Read the model definition and answer for the solid it produces. Units are mm, in the model's axes. Face numbers are marked on the shaded views. A direction names the side the tool comes from. Give positions to 0.01 mm unless a question says otherwise; leave off trailing zeros. Order: outer loops, then holes, each group sorted by start corner. A loop starts at its lowest first (then second) coordinate and runs counter-clockwise, first axis right, second up. Notation, with made-up numbers: (-17.5, 25) - (-5.5, 25) arc R24 cw to (-5.5, 42) - close; hole circle Ø3 at (39, 7.5). An arc over 180 degrees is marked (long way). Use a Markdown table: item, result. Add a question column.
1. Which of the six approach directions +Z, -Z, +X, -X, +Y, -Y give full straight-line access (tool end or side, diameter ignored) to the marked faces 1, 2, 3 and 4?
2. A cutting plane is placed at C-C on y = -30. Determine the outline of the cut face in (x, z), and give its area (3 significant figures).
3. A cutting plane is placed at A-A on x = 0. Determine the outline of the cut face in (y, z).
4. Flat-ended cylindrical pins translate along their axes: P1, Ø15, axis at y = -44, z = 15.5, coming from the +X side; P2, Ø24, axis at x = -49.5, y = -37.5, coming from the +Z side; P3, Ø24, axis at y = -34, z = 13, coming from the -X side; P4, Ø4, axis at x = -16, z = 19, coming from the +Y side. Find the tip coordinate at first contact, or state that the pin passes through.
5. For a pull along Y with two mould halves and no side action, classify the marked faces 5, 6 and 7 as released by +Y, released by -Y, zero draft, split by the parting line, or undercut.
6. Consider L1, parallel to X at y = -50, z = 5; L2, parallel to Y at x = -32.5, z = 25; L3, parallel to Y at x = 9.5, z = -2.5. Determine where each line is inside the solid, lowest interval first.
7. A cutting plane is placed at B-B on z = 5. Determine the outline of the cut face in (x, y), and give its area (3 significant figures).
8. A cutting plane is placed at D-D on y = -17.5. Determine the outline of the cut face in (x, z).
```python
from build123d import *

# Parameters (mm, degrees)
F1_DEPTH = 60
F2_W     = 30
F2_H     = 30
F3_DEPTH = 45
F5_DEPTH = 15.001
F7_DEPTH = 15.001
F8_R     = 20
F9_DEPTH = 60.001


with BuildPart() as f1:
    # F0 (on Front) → F1 (new body)
    with BuildSketch(Plane.XZ):
        with BuildLine():
            Line((60, 30), (-60, 30))
            Line((-60, 30), (-60, -30))
            Line((-60, -30), (-5, -30))
            Line((-5, -30), (-5, -4.434966))
            ThreePointArc((-5, -4.434966), (0, 15.677948), (5, -4.434966))
            Line((5, -4.434966), (5, -30))
            Line((5, -30), (60, -30))
            Line((60, -30), (60, 30))
        make_face()
    extrude(amount=F1_DEPTH)

    # F2 (on face) → F3 (cut)
    with BuildSketch(Plane.XZ.offset(60)):
        with Locations((-45, 15)):
            Rectangle(F2_W, F2_H)
        with Locations((45, 15)):
            Rectangle(F2_W, F2_H)
    extrude(amount=-F3_DEPTH, mode=Mode.SUBTRACT)

    # F4 (on face) → F5 (cut, through all)
    with BuildSketch(Plane.XZ.offset(15)):
        Polygon((-60, 0), (-30, 30), (-60, 30), align=None)
    extrude(amount=-F5_DEPTH, mode=Mode.SUBTRACT)

    # F6 (on face) → F7 (cut, through all)
    with BuildSketch(Plane.XZ.offset(15)):
        Polygon((60, 30), (30, 30), (60, 0), align=None)
    extrude(amount=-F7_DEPTH, mode=Mode.SUBTRACT)

    # F8 (on face) → F9 (cut, through all)
    with BuildSketch(Plane.XY.offset(30)):
        with Locations((0, -30)):
            Circle(F8_R)
    extrude(amount=-F9_DEPTH, mode=Mode.SUBTRACT)


solid = f1.part
```
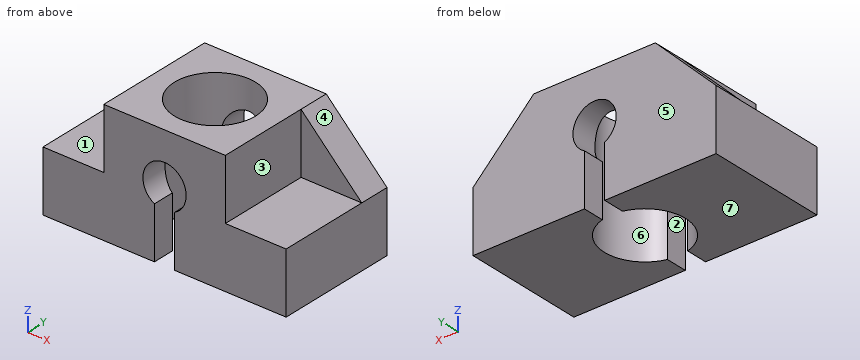
Output values:
| question | item | result |
|---|---|---|
| 1 | face 1 | +Z, -X, -Y |
| 1 | face 2 | -Z, +Y, -Y |
| 1 | face 3 | +Z, +X, -Y |
| 1 | face 4 | +Z, +X, +Y, -Y |
| 2 | outline | (-60, -30) - (-20, -30) - (-20, 30) - (-30, 30) - (-30, 0) - (-60, 0) - close; (20, -30) - (60, -30) - (60, 0) - (30, 0) - (30, 30) - (20, 30) - close |
| 2 | area | 3,000 mm² |
| 3 | outline | (-60, 15.68) - (-50, 15.68) - (-50, 30) - (-60, 30) - close; (-10, 15.68) - (0, 15.68) - (0, 30) - (-10, 30) - close |
| 4 | P1 | x = 30 |
| 4 | P2 | z = 0 |
| 4 | P3 | x = -30 |
| 4 | P4 | y = 0 |
| 5 | face 5 | released by +Y |
| 5 | face 6 | undercut |
| 5 | face 7 | zero draft |
| 6 | L1 | -30 to -10.68, 10.68 to 30 |
| 6 | L2 | -15 to 0 |
| 6 | L3 | -60 to -47.6, -12.4 to 0 |
| 7 | outline | (-55, -15) - (-30, -15) - (-30, -60) - (-10.68, -60) - (-10.68, -46.91) arc R20 cw to (-10.68, -13.09) - (-10.68, 0) - (-55, 0) - close; (10.68, -60) - (30, -60) - (30, -15) - (55, -15) - (55, 0) - (10.68, 0) - (10.68, -13.09) arc R20 cw to (10.68, -46.91) - close |
| 7 | area | 2,620 mm² |
| 8 | outline | (-60, -30) - (-15.61, -30) - (-15.61, 30) - (-30, 30) - (-30, 0) - (-60, 0) - close; (15.61, -30) - (60, -30) - (60, 0) - (30, 0) - (30, 30) - (15.61, 30) - close |
